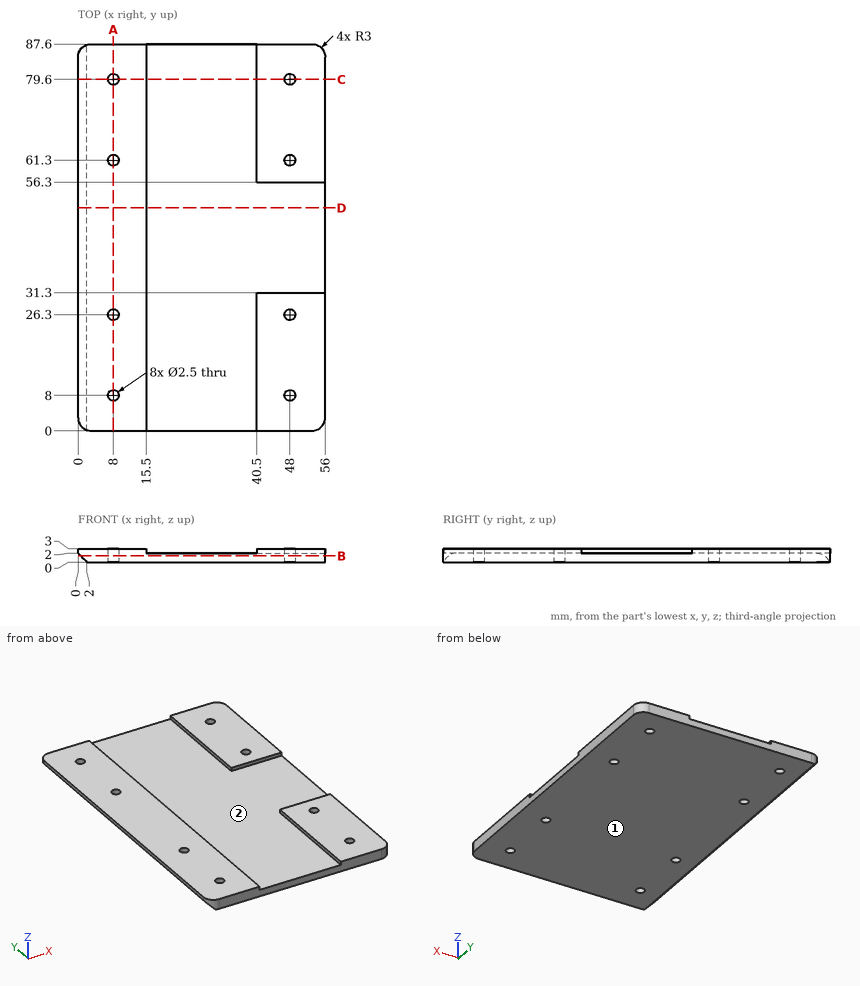
Could you check a few things on this drawing? It's one solid part, dimensions in mm from its lowest x, y, z. A direction names the side the tool comes from. Give positions to 0.01 mm unless a question says otherwise; leave off trailing zeros. Order: outer loops, then holes, each group sorted by start corner. A loop starts at its lowest first (then second) coordinate and runs counter-clockwise, first axis right, second up. Notation, with made-up numbers: (84.5, 50.5) - (110.5, 50.5) arc R30 ccw to (110.5, 88.5) - close; hole circle Ø2 at (-4, 23.5). An arc over 180 degrees is marked (long way). One line per question, with ' | ' between items. Start each with the question number.
Item 1: I want a section at C-C on y = 79.6. Write out the boundary of the cut face in (x, z).
Item 2: I want a section at B-B on z = 1.4. Give the number of separate pieces and of enclosed holes in the cut face, then the cut area to 3 significant figures.
Item 3: I need wall thicknesses on probe 1 along Y at (x, z) = (8, 0.7); probe 2 along Y at (x, z) = (45, 2.65); probe 3 along X at (y, z) = (25, 2.3). Which ranges of each line are inside material? Lowest first, please. Write a range as [from, to].
Item 4: I'm going to push flat-ended pins straight in: pin 1 Ø1.5 at (x, y) = (48, 61.3) entering from +Z; pin 2 Ø1 at (y, z) = (58, 1) entering from -X. Where does each tip first touch, or does it pass through?
Item 5: For the marked faces 1 and 2, which set-ups out of +Z, -Z, +X, -X, +Y, -Y let a thin tool reach every point of the face, with its end or its side?
Item 6: I want a section at D-D on y = 50.5. Write out the boundary of the cut face in (x, z), then the cut area to 4 significant figures.
Item 7: I want a section at A-A on x = 8. Write out the boundary of the cut face in (y, z).
Verdict:
1) outline: (0, 2) - (2, 0) - (6.75, 0) - (6.75, 3) - (0, 3) - close; (9.25, 0) - (46.75, 0) - (46.75, 3) - (40.5, 3) - (40.5, 2) - (15.5, 2) - (15.5, 3) - (9.25, 3) - close; (49.25, 0) - (56, 0) - (56, 3) - (49.25, 3) - close
2) separate pieces: 1 | enclosed holes: 8 | area: 4,810 mm^2
3) probe 1: [0, 6.75], [9.25, 25.05], [27.55, 60.05], [62.55, 78.35], [80.85, 87.6] | probe 2: [0, 31.3], [56.3, 87.6] | probe 3: [0, 15.5], [40.5, 56]
4) pin 1: through | pin 2: x = 0.5
5) face 1: -Z, +X, -X, +Y, -Y | face 2: +Z
6) outline: (0, 2) - (2, 0) - (56, 0) - (56, 2) - (15.5, 2) - (15.5, 3) - (0, 3) - close | area: 125.5 mm^2
7) outline: (0, 0) - (6.75, 0) - (6.75, 3) - (0, 3) - close; (9.25, 0) - (25.05, 0) - (25.05, 3) - (9.25, 3) - close; (27.55, 0) - (60.05, 0) - (60.05, 3) - (27.55, 3) - close; (62.55, 0) - (78.35, 0) - (78.35, 3) - (62.55, 3) - close; (80.85, 0) - (87.6, 0) - (87.6, 3) - (80.85, 3) - close
